The listing builds one solid part. Answer for the finished solid, in the listing's coordinates (mm). Face numbers are marked on the shaded views. A direction names the side the tool comes from. Give positions to 0.01 mm unless a question says otherwise; leave off trailing zeros. Loops run counter-clockwise (first coordinate to the right, second up) from the corner with the lowest first, then second, coordinate; pieces in that order, holes last. Notation, with made-up numbers: M -34,40.5 L -12,40.5 A22 cw -12,66.5 Z; hole C -35,63.25 d5. An arc over 180 degrees is marked long. Use one line per item in the form item = value. Start each with the question number.
1. The part is cut by section D-D (x = -6.75). Write down the section's boundary in (y, z).
2. The mould has two halves that part along X. Classify the marked faces 3, 4 and 5: released by +X, released by -X, zero draft, split by the parting line, or undercut.
3. Each of these flat-tipped pins is pushed along its axis until it touches: pin 1 Ø5.5 at (x, y) = (8.11, -6.7) entering from -Z; pin 2 Ø4 at (x, y) = (-9, 1.5) entering from +Z; pin 3 Ø2 at (y, z) = (-2.5, 1.5) entering from +X. Where does it stop, or does it pass through?
4. The part is cut by section A-A (x = 0). Write down the section's boundary in (y, z).
5. The part is cut by section C-C (z = 10). Write down the section's boundary in (x, y), and give its area (3 significant figures).
6. The part is cut by section B-B (y = -6.7). Write down the section's boundary in (x, z) (1 decimal).
7. For the marked faces 1 and 2, determine the directions among +Z, -Z, +X, -X, +Y, -Y from which every point of the face is accessible in a straight line to the end or side of a thin tool.
8. Straight lines are drawn through the part: line 1 (X direction, y = -4.25, z = -12); line 2 (Z direction, x = 1.5, y = 5.75); line 3 (X direction, y = -7.5, z = -11.5). For each, find the intervals that lie inside material, in ascending order. Write a range as from..to.
from build123d import *

# Parameters (mm, degrees)
BOSS_EXTRUDE1_DEPTH      = 12.7
BOSS_EXTRUDE1_DEPTH_BACK = 12.7
SKETCH1_R                = 11.1125
SKETCH2_R                = 3
CUT_EXTRUDE1_DEPTH       = 7


with BuildPart() as part:
    # Sketch1 → Boss-Extrude1 (new, two sides: drawn at the far end of the back side and taken through both)
    with BuildSketch(Plane(origin=(0, 0, 0), x_dir=(1, 0, 0), z_dir=(0, 1, 0)).offset(-BOSS_EXTRUDE1_DEPTH_BACK)):
        with BuildLine():
            Line((-14.1125, 0), (-14.1125, 14.1125))
            Line((-14.1125, 14.1125), (-14.1125, 18.1125))
            Line((-14.1125, 18.1125), (14.1125, 18.1125))
            Line((14.1125, 18.1125), (14.1125, 14.1125))
            Line((14.1125, 14.1125), (14.1125, 0))
            ThreePointArc((14.1125, 0), (0, -14.1125), (-14.1125, 0))
        make_face()
        with Locations(Location((0, 0, 0), (0, 0, 270))):
            Circle(SKETCH1_R, mode=Mode.SUBTRACT)
    extrude(amount=BOSS_EXTRUDE1_DEPTH + BOSS_EXTRUDE1_DEPTH_BACK)

    # Sketch2 → Cut-Extrude1 (cut)
    with BuildSketch(Plane(origin=(0, 0, -18.1125), x_dir=(-1, 0, 0), z_dir=(0, 0, -1))):
        with Locations((8.1125, -6.7)):
            Circle(SKETCH2_R)
        with Locations((-8.1125, -6.7)):
            Circle(SKETCH2_R)
        with Locations((-8.1125, 6.7)):
            Circle(SKETCH2_R)
        with Locations((8.1125, 6.7)):
            Circle(SKETCH2_R)
    extrude(amount=-CUT_EXTRUDE1_DEPTH, mode=Mode.SUBTRACT)


solid = part.part
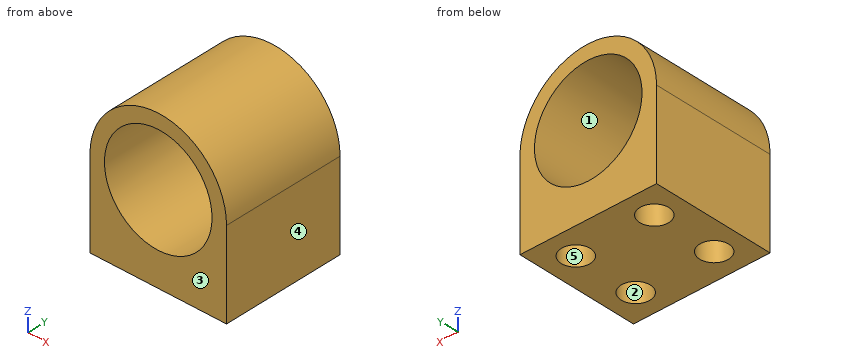
Derived:
q1.outline = M -12.7,-18.11 L -9.37,-18.11 L -9.37,-11.11 L -4.03,-11.11 L -4.03,-18.11 L 4.03,-18.11 L 4.03,-11.11 L 9.37,-11.11 L 9.37,-18.11 L 12.7,-18.11 L 12.7,-8.83 L -12.7,-8.83 Z; M -12.7,8.83 L 12.7,8.83 L 12.7,12.39 L -12.7,12.39 Z
q2.face_3 = zero draft
q2.face_4 = released by +X
q2.face_5 = undercut
q3.pin_1 = -11.11
q3.pin_2 = 12.25
q3.pin_3 = 14.1
q4.outline = M -12.7,-18.11 L 12.7,-18.11 L 12.7,-11.11 L -12.7,-11.11 Z; M -12.7,11.11 L 12.7,11.11 L 12.7,14.11 L -12.7,14.11 Z
q5.outline = M -9.96,-12.7 L -4.85,-12.7 L -4.85,12.7 L -9.96,12.7 Z; M 4.85,-12.7 L 9.96,-12.7 L 9.96,12.7 L 4.85,12.7 Z
q5.area = 260 mm2
q6.outline = M -14.1,-18.1 L -11.1,-18.1 L -11.1,-11.1 L -5.1,-11.1 L -5.1,-18.1 L 5.1,-18.1 L 5.1,-11.1 L 11.1,-11.1 L 11.1,-18.1 L 14.1,-18.1 L 14.1,0 A14.1 ccw -14.1,0 Z; hole C 0,0 d22.2
q7.face_1 = +Y, -Y
q7.face_2 = -Z
q8.line_1 = -14.11..-9.84, -6.38..6.38, 9.84..14.11
q8.line_2 = -18.11..-11.01, 11.01..14.03
q8.line_3 = -14.11..-11, -5.22..5.22, 11..14.11
